from build123d import *

# Parameters (mm, degrees)
F0_R     = 11.2
F1_DEPTH = 7


# Not quite as in the source:
# - a feature names something its author has since deleted; it is built from what else it names


with BuildPart() as f1:
    # F0 (on Front) → F1 (new body)
    with BuildSketch(Plane.XZ):
        with BuildLine():
            Line((-23.5628467053, 13.316613622), (-6.9041872543, 13.316613622))
            ThreePointArc((-6.9041872543, 13.316613622), (-15, 0), (-6.9041872543, -13.316613622))
            Line((-6.9041872543, -13.316613622), (-23.5628467053, -13.316613622))
            Line((-23.5628467053, -13.316613622), (-23.5628467053, -21.1474765092))
            Line((-23.5628467053, -21.1474765092), (0, -21.1474765092))
            Line((0, -21.1474765092), (23.5628467053, -21.1474765092))
            Line((23.5628467053, -21.1474765092), (23.5628467053, -13.316613622))
            Line((23.5628467053, -13.316613622), (6.9041872543, -13.316613622))
            ThreePointArc((6.9041872543, -13.316613622), (15, 0), (6.9041872543, 13.316613622))
            Line((6.9041872543, 13.316613622), (23.5628467053, 13.316613622))
            Line((23.5628467053, 13.316613622), (23.5628467053, 21.1474765092))
            Line((23.5628467053, 21.1474765092), (0, 21.1474765092))
            Line((0, 21.1474765092), (-23.5628467053, 21.1474765092))
            Line((-23.5628467053, 21.1474765092), (-23.5628467053, 13.316613622))
        make_face()
        Circle(F0_R, mode=Mode.SUBTRACT)
    extrude(amount=F1_DEPTH)


solid = f1.part
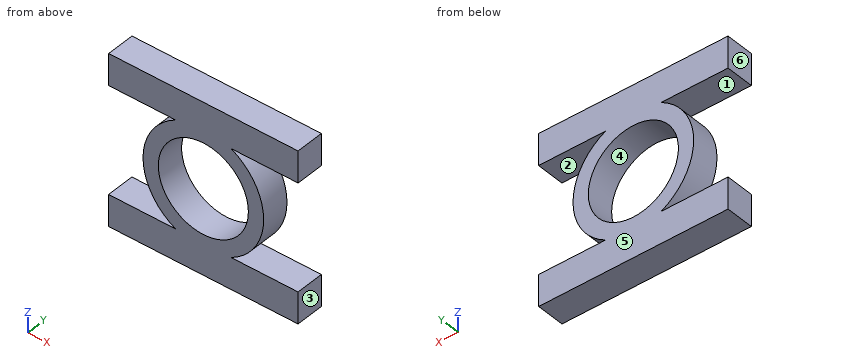
Source: CAD feature listing. Evaluate the final solid. Frame: model axes, mm. Face numbers are marked on the shaded views. A direction names the side the tool comes from. Give positions to 0.01 mm unless a question says otherwise; leave off trailing zeros. Write each loop counter-clockwise with the first axis right and the second up, starting at its lowest first coordinate (ties: lowest second). Pieces come first, ordered by that corner, then holes. Notation, with made-up numbers: (79, -4) -> (119, -4) arc R7 cw to (119, 2) -> close; hole circle Ø7 at (54, 38). An arc over 180 degrees is marked (long way). Write item = value, one per line.
Q1. Cut plane B-B on x = 13.5. Return loops of the section in (y, z), then the cut area to 3 significant figures.
Here are the results:
outline = (-7, -21.15) -> (0, -21.15) -> (0, -13.32) -> (-7, -13.32) -> close; (-7, -6.54) -> (0, -6.54) -> (0, 6.54) -> (-7, 6.54) -> close; (-7, 13.32) -> (0, 13.32) -> (0, 21.15) -> (-7, 21.15) -> close
area = 201 mm²
Q2. Cut plane A-A on z = 0. Return loops of the section in (x, y), then the cut area to 3 significant figures.
Here are the results:
outline = (-15, -7) -> (-11.2, -7) -> (-11.2, 0) -> (-15, 0) -> close; (11.2, -7) -> (15, -7) -> (15, 0) -> (11.2, 0) -> close
area = 53.2 mm²
Q3. Cut plane D-D on x = 0. Return loops of the section in (y, z), then the cut area to 3 significant figures.
Here are the results:
outline = (-7, -21.15) -> (0, -21.15) -> (0, -11.2) -> (-7, -11.2) -> close; (-7, 11.2) -> (0, 11.2) -> (0, 21.15) -> (-7, 21.15) -> close
area = 139 mm²
Q4. Cut plane C-C on y = -4.75. Return loops of the section in (x, z), then the cut area to 3 significant figures.
Here are the results:
outline = (-23.56, -21.15) -> (23.56, -21.15) -> (23.56, -13.32) -> (6.9, -13.32) arc R15 ccw to (6.9, 13.32) -> (23.56, 13.32) -> (23.56, 21.15) -> (-23.56, 21.15) -> (-23.56, 13.32) -> (-6.9, 13.32) arc R15 ccw to (-6.9, -13.32) -> (-23.56, -13.32) -> close; hole circle Ø22.4 at (0, 0)
area = 1,020 mm²
Q5. Mould query, pull axis X, two halves, no side actions, for the marked faces 4, 5 and 6. Classes: +X half, -X half, draft (parallel to the pull), parting line (faces both ways), or undercut.
Here are the results:
face_4 = undercut
face_5 = draft
face_6 = -X half
Q6. Line query: line 1 (Z direction, x = 0, y = -1.25); line 2 (Z direction, x = -8, y = -3.25); line 3 (Z direction, x = -20, y = -1.5). Output: solid intervals per line, ascending. Write a range as from..to.
Here are the results:
line_1 = -21.15..-11.2, 11.2..21.15
line_2 = -21.15..-13.32, -12.69..-7.84, 7.84..12.69, 13.32..21.15
line_3 = -21.15..-13.32, 13.32..21.15
Q7. Reachability of the marked faces 1, 2 and 3 from +Z, -Z, +X, -X, +Y, -Y: full face, straight path, thin tool, end or side. Return the list, or none.
Here are the results:
face_1 = -X, +Y, -Y
face_2 = +X, +Y, -Y
face_3 = +Z, -Z, +X, +Y, -Y
Q8. First-contact query: pin 1 (1.5 mm diameter, centred on x = -5, z = -16.5, fed in from +Y). Flat tip, straight axial feed; report the tip coordinate or a pass-through.
Here are the results:
pin_1 = 0
